The model under review builds one solid part; all positions refer to its coordinate system, in mm. Face numbers are marked on the shaded views. A direction names the side the tool comes from. Coordinates: 2 decimals unless noted, no trailing zeros. Order: outer loops, then holes, each group sorted by start corner. A loop starts at its lowest first (then second) coordinate and runs counter-clockwise, first axis right, second up. Notation, with made-up numbers: M 7.5,67.5 L 46.5,67.5 A12 ccw 46.5,86.5 Z; hole C 46.25,-27.5 d10. An arc over 180 degrees is marked long. Write each question's results on one line, items separated by ' | '.
from build123d import *

# Parameters (mm, degrees)
SKETCH1_W            = 101.6
SKETCH1_H            = 25.4
BOSS_EXTRUDE1_DEPTH  = 3.175
BOSS_EXTRUDE2_DEPTH  = 6.35
SKETCH4_W            = 6.35
SKETCH4_H            = 2.54
CUT_EXTRUDE2_DEPTH   = 1.27
FILLET2_R            = 0.254
FILLET3_R            = 0.254
FILLET2_OF_MIRROR4_R = 0.254
FILLET3_OF_MIRROR4_R = 0.254
SKETCH6_W            = 7.62
SKETCH6_H            = 25.4
BOSS_EXTRUDE4_DEPTH  = 2.54
CUT_EXTRUDE3_REACH   = 21.05
SKETCH7_W            = 92.71
SKETCH7_H            = 20.32
CUT_EXTRUDE4_REACH   = 103.6
SKETCH8_R            = 1.27


with BuildPart() as part:
    # Sketch1 → Boss-Extrude1 (new body, symmetric)
    with BuildSketch(Plane.XY):
        with Locations((50.8, 0)):
            Rectangle(SKETCH1_W, SKETCH1_H)
    extrude(amount=BOSS_EXTRUDE1_DEPTH, both=True)

    # Sketch2 → Boss-Extrude2 (add)
    with BuildSketch(Plane.ZY.offset(-12.7)):
        Polygon((-3.175, 12.7), (-15.875, 12.7), (-15.875, -12.7), (-3.175, -12.7), (-3.175, -10.16), (-13.335, -10.16), (-13.335, 10.16), (-3.175, 10.16), align=None)
    boss_extrude2 = extrude(amount=BOSS_EXTRUDE2_DEPTH)

    # Sketch4 → Cut-Extrude2 (cut)
    with BuildSketch(Plane.XY.offset(-13.335)):
        with Locations((9.525, 0)):
            Rectangle(SKETCH4_W, SKETCH4_H)
    cut_extrude2 = extrude(amount=-CUT_EXTRUDE2_DEPTH, mode=Mode.SUBTRACT)

    # Fillet2
    fillet2_edges = [part.edges().sort_by_distance(p)[0] for p in [
        (6.35, 0, -14.605),
        (6.35, -1.27, -13.97),
        (6.35, 1.27, -13.97),
    ]]
    fillet(fillet2_edges, radius=FILLET2_R)

    # Fillet3
    fillet3_edges = [part.edges().sort_by_distance(p)[0] for p in [
        (12.7, 0, -14.605),
        (12.7, 1.27, -13.97),
        (12.7, -1.27, -13.97),
    ]]
    fillet(fillet3_edges, radius=FILLET3_R)

    # Mirror4: Boss-Extrude2, Cut-Extrude2 across plane
    add(boss_extrude2.mirror(Plane.XY))
    add(cut_extrude2.mirror(Plane.XY), mode=Mode.SUBTRACT)

    # Fillet2 of Mirror4
    fillet2_of_mirror4_edges = [part.edges().sort_by_distance(p)[0] for p in [
        (6.35, 0, 14.605),
        (6.35, -1.27, 13.97),
        (6.35, 1.27, 13.97),
    ]]
    fillet(fillet2_of_mirror4_edges, radius=FILLET2_OF_MIRROR4_R)

    # Fillet3 of Mirror4
    fillet3_of_mirror4_edges = [part.edges().sort_by_distance(p)[0] for p in [
        (12.7, 0, 14.605),
        (12.7, 1.27, 13.97),
        (12.7, -1.27, 13.97),
    ]]
    fillet(fillet3_of_mirror4_edges, radius=FILLET3_OF_MIRROR4_R)

    # Sketch6 → Boss-Extrude4 (add)
    with BuildSketch(Plane(origin=(101.6, 0, 0), x_dir=(0, 0, -1), z_dir=(1, 0, 0))):
        with Locations((6.985, 0)):
            Rectangle(SKETCH6_W, SKETCH6_H)
    boss_extrude4 = extrude(amount=-BOSS_EXTRUDE4_DEPTH)

    # Mirror5: Boss-Extrude4 across plane
    add(boss_extrude4.mirror(Plane.XY))

    # Sketch7 → Cut-Extrude3 (cut, up to next)
    with BuildSketch(Plane.XY.offset(3.175), mode=Mode.PRIVATE) as cut_extrude3_sk1:
        with Locations((52.705, 0)):
            Rectangle(SKETCH7_W, SKETCH7_H)
    cut_extrude3_tool1 = extrude(cut_extrude3_sk1.sketch, amount=-CUT_EXTRUDE3_REACH, mode=Mode.PRIVATE) & part.part
    add(cut_extrude3_tool1.solids().sort_by_distance((52.705, 0, 3.175))[0], mode=Mode.SUBTRACT)

    # Sketch8 → Cut-Extrude4 (cut, up to next)
    with BuildSketch(Plane.ZY, mode=Mode.PRIVATE) as cut_extrude4_sk1:
        Circle(SKETCH8_R)
    cut_extrude4_tool1 = extrude(cut_extrude4_sk1.sketch, amount=-CUT_EXTRUDE4_REACH, mode=Mode.PRIVATE) & part.part
    add(cut_extrude4_tool1.solids().sort_by_distance((0, 0, 0))[0], mode=Mode.SUBTRACT)


solid = part.part
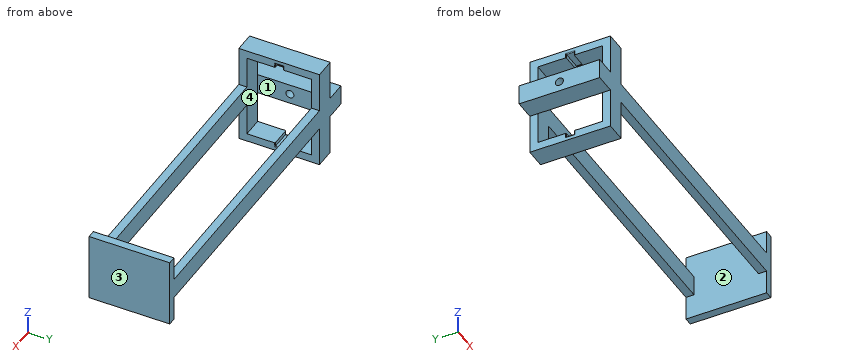
1) The part is to be moulded in two halves that separate along Z. For the marked faces 1 and 2, say which applies: pulls with the +Z half, pulls with the -Z half, needs draft (parallel to the pull), parting line crosses it, or undercut.
Solutions:
face 1: undercut | face 2: needs draft
2) Take a section at D-D on x = 8.5. State the section outline as (y, z) points (3 decimals), plus the area to 3 significant figures.
Solutions:
outline: M -12.7,-15.875 L 12.7,-15.875 L 12.7,15.875 L -12.7,15.875 Z; hole M -10.16,-13.335 L -1.27,-13.335 L -1.27,-14.605 L 1.27,-14.605 L 1.27,-13.335 L 10.16,-13.335 L 10.16,13.335 L 1.27,13.335 L 1.27,14.605 L -1.27,14.605 L -1.27,13.335 L -10.16,13.335 Z | area: 258 mm2
3) To check wall thickness, follow line 1 along Y through (x, z) = (3.5, 0); line 2 along X through (y, z) = (1.5, -2); line 3 along X through (y, z) = (11, 8.5). State the ranges of each line that lie inside material, in increasing order.
Solutions:
line 1: -12.7 to -1.27, 1.27 to 12.7 | line 2: 0 to 6.35, 99.06 to 101.6 | line 3: 6.35 to 12.7, 99.06 to 101.6
4) Take a section at B-B on y = 4.5. State the section outline as (x, z) points (3 decimals).
Solutions:
outline: M 0,-3.175 L 6.35,-3.175 L 6.35,3.175 L 0,3.175 Z; M 6.35,-15.875 L 12.7,-15.875 L 12.7,-13.335 L 6.35,-13.335 Z; M 6.35,13.335 L 12.7,13.335 L 12.7,15.875 L 6.35,15.875 Z; M 99.06,-10.795 L 101.6,-10.795 L 101.6,10.795 L 99.06,10.795 Z
5) For the marked faces 3 and 4, list the 3-axis set-ups (+Z, -Z, +X, -X, +Y, -Y) from which the entire face can be reached by the end or side of a thin tool; tool diameter is ignored.
Solutions:
face 3: +Z, -Z, +X, +Y, -Y | face 4: none
6) Take a section at C-C on z = -7.5. State the section outline as (x, y) points, plus the area to 3 significant figures.
Solutions:
outline: M 6.35,-12.7 L 12.7,-12.7 L 12.7,-10.16 L 6.35,-10.16 Z; M 6.35,10.16 L 12.7,10.16 L 12.7,12.7 L 6.35,12.7 Z; M 99.06,-12.7 L 101.6,-12.7 L 101.6,12.7 L 99.06,12.7 Z | area: 96.8 mm2
7) Take a section at A-A on x = 77.5. State the section outline as (y, z) points (3 decimals).
Solutions:
outline: M -12.7,-3.175 L -10.16,-3.175 L -10.16,3.175 L -12.7,3.175 Z; M 10.16,-3.175 L 12.7,-3.175 L 12.7,3.175 L 10.16,3.175 Z
8) For pin 1 (0.8 mm diameter, centred on x = 100, y = -6, fed in from +Z) (3 decimals); pin 2 (10 mm diameter, centred on y = -5, z = 11.5, fed in from -X); pin 3 (3 mm diameter, centred on x = 89, z = -3.5, fed in from +Y); pin 4 (0.8 mm diameter, centred on x = 61.5, y = 11.5, fed in from -Z) (3 decimals), all flat-tipped, find the tip position at first contact; note any pin that passes through.
Solutions:
pin 1: z = 10.795 | pin 2: x = 6.35 | pin 3: y = 12.7 | pin 4: z = -3.175
